Here's the drawing with two shaded views (mm, measured from the low corner). I have some questions. A direction names the side the tool comes from. Give positions to 0.01 mm unless a question says otherwise; leave off trailing zeros. Loops run counter-clockwise (first coordinate to the right, second up) from the corner with the lowest first, then second, coordinate; pieces in that order, holes last. Notation, with made-up numbers: (62, -11) -> (90, -11) arc R28 ccw to (90, 23) -> close; hole circle Ø3 at (67, 60). An arc over 180 degrees is marked (long way). Put each result on its own line as item: value.
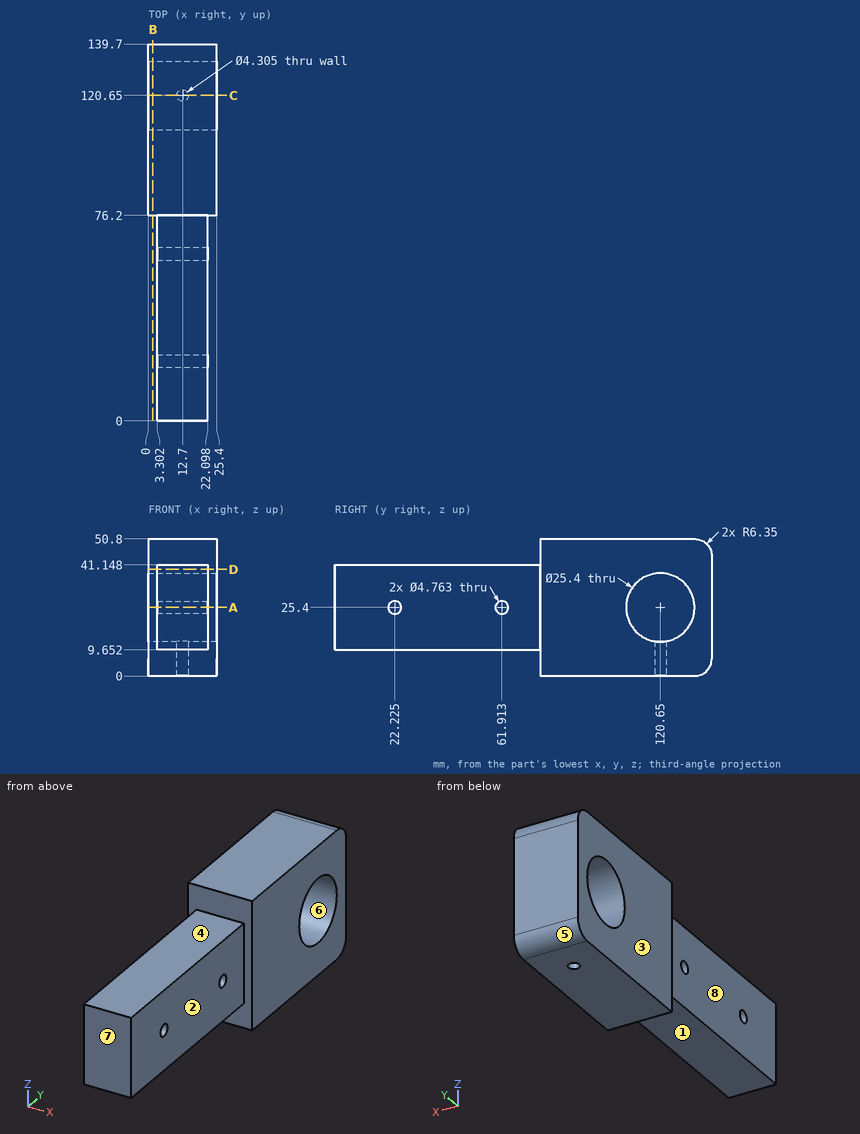
1. If we section it at A-A (z = 25.4): List the corners of the cut face in (x, y) for me, then the cut area to 3 significant figures.
Recorded:
outline: (0, 76.2) -> (3.3, 76.2) -> (3.3, 64.29) -> (22.1, 64.29) -> (22.1, 76.2) -> (25.4, 76.2) -> (25.4, 107.95) -> (0, 107.95) -> close; (0, 133.35) -> (25.4, 133.35) -> (25.4, 139.7) -> (0, 139.7) -> close; (3.3, 0) -> (22.1, 0) -> (22.1, 19.84) -> (3.3, 19.84) -> close; (3.3, 24.61) -> (22.1, 24.61) -> (22.1, 59.53) -> (3.3, 59.53) -> close
area: 2,220 mm^2
2. I need wall thicknesses on line 1 (Y direction, x = 15.5, z = 25.4); line 2 (X direction, y = 120.65, z = 3.25); line 3 (Y direction, x = 10.5, z = 26) (1 decimal). Which ranges of each line are inside material? Lowest first, please.
Recorded:
line 1: y = 0 to 19.84, 24.61 to 59.53, 64.29 to 107.95, 133.35 to 139.7
line 2: x = 0 to 10.55, 14.85 to 25.4
line 3: y = 0 to 19.9, 24.5 to 59.6, 64.2 to 108, 133.3 to 139.7
3. If we section it at D-D (z = 39.5): List the corners of the cut face in (x, y) for me, then the cut area to 4 significant figures.
Recorded:
outline: (0, 76.2) -> (3.3, 76.2) -> (3.3, 0) -> (22.1, 0) -> (22.1, 76.2) -> (25.4, 76.2) -> (25.4, 139.7) -> (0, 139.7) -> close
area: 3,045 mm^2
4. For the marked faces 1, 2, 3 and 4, which set-ups out of +Z, -Z, +X, -X, +Y, -Y let a thin tool reach every point of the face, with its end or its side?
Recorded:
face 1: -Z, +X, -X, -Y
face 2: +Z, -Z, +X, -Y
face 3: +Z, -Z, -X, +Y, -Y
face 4: +Z, +X, -X, -Y
5. Thinking about a two-plate mould opening in Y: for the marked faces 5, 6, 7 and 8, which applies, pulls with the +Y half, pulls with the -Y half, needs draft (parallel to the pull), parting line crosses it, or undercut?
Recorded:
face 5: pulls with the +Y half
face 6: undercut
face 7: pulls with the -Y half
face 8: needs draft
6. If we section it at C-C (y = 120.65): List the corners of the cut face in (x, z) for me.
Recorded:
outline: (0, 0) -> (10.55, 0) -> (10.55, 12.7) -> (0, 12.7) -> close; (0, 38.1) -> (25.4, 38.1) -> (25.4, 50.8) -> (0, 50.8) -> close; (14.85, 0) -> (25.4, 0) -> (25.4, 12.7) -> (14.85, 12.7) -> close
7. If we section it at B-B (x = 1.75): List the corners of the cut face in (y, z) for me.
Recorded:
outline: (76.2, 0) -> (133.35, 0) arc R6.35 ccw to (139.7, 6.35) -> (139.7, 44.45) arc R6.35 ccw to (133.35, 50.8) -> (76.2, 50.8) -> close; hole circle Ø25.4 at (120.65, 25.4)
8. I'm going to push flat-ended pins straight in: pin 1 (15 mm diameter, centred on x = 14.5, y = 35.5, fed in from +Z); pin 2 (2.5 mm diameter, centred on x = 12.7, y = 120.65, fed in from -Z); pin 3 (4.5 mm diameter, centred on y = 61.91, z = 25.4, fed in from +X); pin 4 (9.5 mm diameter, centred on x = 15.5, y = 49, fed in from -Z). Where does each tip first touch, or does it pass through?
Recorded:
pin 1: stops at z = 41.15
pin 2: stops at z = 38.04
pin 3: passes through
pin 4: stops at z = 9.65
